from build123d import *

# Parameters (mm, degrees)
ESQUISSE1_W                  = 340
ESQUISSE1_H                  = 100.00000000000001
BOSS_EXTRU_1_DEPTH           = 10
ENL_V_MAT_EXTRU_1_DEPTH      = 355.54195802471673
ENL_V_MAT_EXTRU_1_DEPTH_BACK = 355.54195802471673
ESQUISSE2_R                  = 3.0000000000000018
ESQUISSE2_R_2                = 6.0000000000000036
ESQUISSE2_R_3                = 5.000000000000005
ESQUISSE2_R_4                = 6.000000000000017
ESQUISSE2_R_5                = 2.9999999999999947
ESQUISSE2_R_6                = 21.000000000000014
ESQUISSE2_W                  = 22.00000000000003
ESQUISSE2_H                  = 20.000000000000007
ENL_V_MAT_EXTRU_2_DEPTH      = 355.54195802471673
ENL_V_MAT_EXTRU_2_DEPTH_BACK = 355.54195802471673
ESQUISSE3_R                  = 2.2500000000000093
ESQUISSE3_R_2                = 2.2499999999999964
ESQUISSE3_R_3                = 2.2500000000000027
ESQUISSE3_R_4                = 2.2500000000000138
ESQUISSE5_R                  = 27.500000000000032
ESQUISSE5_R_2                = 8.999999999999984
ESQUISSE5_R_3                = 7.5000000000000115
ESQUISSE5_R_4                = 18.99999999999999
ESQUISSE5_R_5                = 11.499999999999993
ESQUISSE5_R_6                = 14.999999999999998
ESQUISSE5_R_7                = 11.499999999999998
ESQUISSE5_R_8                = 10.5
ENL_V_MAT_EXTRU_3_DEPTH      = 8
ESQUISSE6_W                  = 5.2500000000000036
ESQUISSE6_H                  = 11.999999999999993
ESQUISSE6_W_2                = 5.250000000000007
ESQUISSE6_W_3                = 5.25
BOSS_EXTRU_2_DEPTH           = 2
ESQUISSE8_R                  = 2.0000000000000027
ESQUISSE8_R_2                = 2.0000000000000018
ESQUISSE8_R_3                = 1.9999999999999967
ENL_V_MAT_EXTRU_4_DEPTH      = 10
ESQUISSE9_R                  = 6.999999999999988
ESQUISSE9_R_2                = 7.000000000000015
ESQUISSE9_R_3                = 7.000000000000002
ENL_V_MAT_EXTRU_5_DEPTH      = 8
CONG_1_R                     = 2
ENL_V_MAT_EXTRU_6_DEPTH      = 355.49118478405074
ENL_V_MAT_EXTRU_6_DEPTH_BACK = 355.49118478405074
CONG_2_R                     = 1.5
CONG_3_R                     = 1


with BuildPart() as part:
    # Esquisse1 → Boss.-Extru.1 (new body)
    with BuildSketch(Plane.XY):
        with Locations((170, 50.00000000000001)):
            Rectangle(ESQUISSE1_W, ESQUISSE1_H)
    extrude(amount=BOSS_EXTRU_1_DEPTH)

    # Esquisse2 → Enlèv. mat.-Extru.1 (cut, two sides: drawn at the far end of the back side and taken through both)
    with BuildSketch(Plane.XY.offset(10).offset(-ENL_V_MAT_EXTRU_1_DEPTH_BACK)):
        with Locations((15.000000000000007, 50)):
            Circle(ESQUISSE2_R)
        with Locations((41.00000000000001, 49.99999999999999)):
            Circle(ESQUISSE2_R_2)
        with Locations((86, 49.99999999999999)):
            Circle(ESQUISSE2_R_3)
        with Locations((131, 50)):
            Circle(ESQUISSE2_R_4)
        with Locations((216.00000000000003, 50)):
            Circle(ESQUISSE2_R_5)
        with Locations((261, 50)):
            Circle(ESQUISSE2_R_5)
        with Locations((306, 50)):
            Circle(ESQUISSE2_R_6)
        with Locations((171, 50)):
            Rectangle(ESQUISSE2_W, ESQUISSE2_H)
    extrude(amount=ENL_V_MAT_EXTRU_1_DEPTH + ENL_V_MAT_EXTRU_1_DEPTH_BACK, mode=Mode.SUBTRACT)

    # Esquisse3 → Enlèv. mat.-Extru.2 (cut, two sides: drawn at the far end of the back side and taken through both)
    with BuildSketch(Plane.XY.offset(10).offset(-ENL_V_MAT_EXTRU_2_DEPTH_BACK)):
        with Locations((170, 80)):
            Circle(ESQUISSE3_R)
        with Locations((100, 80)):
            Circle(ESQUISSE3_R_2)
        with Locations((30, 80)):
            Circle(ESQUISSE3_R_3)
        with Locations(Location((310.00000000000006, 80, 0), (0, 0, 180))):
            Circle(ESQUISSE3_R_4)
        with Locations(Location((240.00000000000003, 80, 0), (0, 0, 180))):
            Circle(ESQUISSE3_R)
    extrude(amount=ENL_V_MAT_EXTRU_2_DEPTH + ENL_V_MAT_EXTRU_2_DEPTH_BACK, mode=Mode.SUBTRACT)

    # Esquisse5 → Enlèv. mat.-Extru.3 (cut)
    with BuildSketch(Plane(origin=(0, 0, 0), x_dir=(-1, 0, 0), z_dir=(0, 0, -1))):
        with Locations((-306, 50)):
            Circle(ESQUISSE5_R)
        with Locations((-261, 50)):
            Circle(ESQUISSE5_R_2)
        with Locations((-216.00000000000003, 50)):
            Circle(ESQUISSE5_R_3)
        with Locations((-171, 50)):
            Circle(ESQUISSE5_R_4)
        with Locations((-131, 50)):
            Circle(ESQUISSE5_R_5)
        with Locations((-86, 49.99999999999999)):
            Circle(ESQUISSE5_R_6)
        with Locations((-41.00000000000001, 49.99999999999999)):
            Circle(ESQUISSE5_R_7)
        with Locations((-15.000000000000007, 50)):
            Circle(ESQUISSE5_R_8)
    extrude(amount=-ENL_V_MAT_EXTRU_3_DEPTH, mode=Mode.SUBTRACT)

    # Esquisse6 → Boss.-Extru.2 (add)
    with BuildSketch(Plane.XY.offset(10)):
        with Locations((33.12500000000001, 50)):
            Rectangle(ESQUISSE6_W, ESQUISSE6_H)
        with Locations((48.875000000000014, 50)):
            Rectangle(ESQUISSE6_W_2, ESQUISSE6_H)
        with Locations((123.12499999999997, 50)):
            Rectangle(ESQUISSE6_W_3, ESQUISSE6_H)
        with Locations((138.87500000000003, 50)):
            Rectangle(ESQUISSE6_W_3, ESQUISSE6_H)
    extrude(amount=-BOSS_EXTRU_2_DEPTH)

    # Esquisse8 → Enlèv. mat.-Extru.4 (cut)
    with BuildSketch(Plane.XY.offset(10)):
        with Locations((5, 90)):
            Circle(ESQUISSE8_R)
        with Locations(Location((5.00000000000001, 10.000000000000009, 0), (0, 0, 180))):
            Circle(ESQUISSE8_R_2)
        with Locations((335, 10.000000000000009)):
            Circle(ESQUISSE8_R_3)
        with Locations(Location((335, 90, 0), (0, 0, 180))):
            Circle(ESQUISSE8_R_3)
    extrude(amount=-ENL_V_MAT_EXTRU_4_DEPTH, mode=Mode.SUBTRACT)

    # Esquisse9 → Enlèv. mat.-Extru.5 (cut)
    with BuildSketch(Plane(origin=(0, 0, 0), x_dir=(-1, 0, 0), z_dir=(0, 0, -1))):
        with Locations((-310.00000000000006, 80)):
            Circle(ESQUISSE9_R)
        with Locations((-240.00000000000003, 80)):
            Circle(ESQUISSE9_R_2)
        with Locations((-170, 80)):
            Circle(ESQUISSE9_R_2)
        with Locations((-100, 80)):
            Circle(ESQUISSE9_R_3)
        with Locations((-30, 80)):
            Circle(ESQUISSE9_R_3)
    extrude(amount=-ENL_V_MAT_EXTRU_5_DEPTH, mode=Mode.SUBTRACT)

    # Congé1
    cong_1_edges = [part.edges().sort_by_distance(p)[0] for p in [
        (303.5061116987467, 77.38668510683382, 4),
        (315.5823162488517, 75.77652450015313, 4),
    ]]
    fillet(cong_1_edges, radius=CONG_1_R)

    # Esquisse10 → Enlèv. mat.-Extru.6 (cut, two sides: drawn at the far end of the back side and taken through both)
    with BuildSketch(Plane(origin=(0, 0, 8), x_dir=(-1, 0, 0), z_dir=(0, 0, -1)).offset(-ENL_V_MAT_EXTRU_6_DEPTH_BACK)):
        Polygon((-314.13172798364525, 65.90990257669736), (-321.90990257669733, 58.13172798364529), (-330.39518395093586, 66.61700935788389), (-322.6170093578838, 74.39518395093592), align=None)
        Polygon((-290.09009742330267, 41.8682720163547), (-281.60481604906414, 33.382990642116134), (-289.3829906421162, 25.60481604906408), (-297.86827201635475, 34.09009742330265), align=None)
    extrude(amount=ENL_V_MAT_EXTRU_6_DEPTH + ENL_V_MAT_EXTRU_6_DEPTH_BACK, mode=Mode.SUBTRACT)

    # Congé2
    cong_2_edges = [part.edges().sort_by_distance(p)[0] for p in [
        (281.60481604906414, 33.382990642116134, 5),
        (295.55817664855954, 31.780002055507403, 9),
        (289.3829906421162, 25.60481604906408, 5),
        (287.78000205550745, 39.55817664855947, 9),
        (330.39518395093586, 66.61700935788389, 5),
        (324.21999794449255, 60.44182335144051, 9),
        (316.44182335144046, 68.21999794449256, 9),
        (322.6170093578838, 74.39518395093592, 5),
    ]]
    fillet(cong_2_edges, radius=CONG_2_R)

    # Congé3
    # the kernel refuses this fillet: 1 mm, written as the material it takes off along each edge
    with BuildSketch(Plane(origin=(328.9416461797837, 65.16347158673169, 8), x_dir=(0.5395485077638712, -0.8419545164495408, 0), z_dir=(0, 0, -1))) as cong_3_piece_1:
        with BuildLine():
            CenterArc((0.7917838484009534, -0.9999000393817246), CONG_3_R, 90.81013186536997, 71.06099512229089)
            Line((-0.15857520364130714, -0.688744656652602), (-0.2536111088455419, -0.6576291183796682))
            ThreePointArc((-0.2536111088455419, -0.6576291183796682), (-0.216495562393325, -0.5213782577373202), (-0.09768701566509973, 0.02138333394130856))
            Line((-0.09768701566509973, 0.02138333394130856), (0.00141389972929694, 0.09999000393815428))
            ThreePointArc((0.00141389972929694, 0.09999000393815428), (0.3888224255540418, 0.09725108299714401), (0.7762309513787835, 0.09999000393816994))
            Line((0.7762309513787835, 0.09999000393816994), (0.7776448511080656, -5e-17))
        make_face()
    extrude(amount=9.944112127770163, mode=Mode.SUBTRACT)
    with BuildSketch(Plane(origin=(321.1634715867316, 72.94164617978372, 8), x_dir=(0.7147000811371469, 0.6994310502276516, 0), z_dir=(0, 0, -1))) as cong_3_piece_2:
        with BuildLine():
            CenterArc((0.7967561378121499, -0.9959424723360712), CONG_3_R, 95.16315700004625, 71.0609951222958)
            Line((-0.17447860578954866, -0.7578184021101204), (-0.27160208014971443, -0.7340059950875214))
            ThreePointArc((-0.27160208014971443, -0.7340059950875214), (-0.18201092031799704, -0.35708917183648514), (-0.09775794201756788, 0.02105670374221132))
            Line((-0.09775794201756788, 0.02105670374221132), (0.00107968352981501, 0.09999417124750024))
            ThreePointArc((0.00107968352981501, 0.09999417124750024), (0.5566601276180686, 0.093995311039016), (0.6977647438705182, 0.09959424723359925))
            Line((0.6977647438705182, 0.09959424723359925), (0.7067639615015904, -4e-17))
        make_face()
    extrude(amount=9.94411212777035, mode=Mode.SUBTRACT)
    with BuildSketch(Plane(origin=(283.0583538202163, 34.836528413268304, 8), x_dir=(-0.6994310502276408, -0.7147000811371573, 0), z_dir=(0, 0, -1))) as cong_3_piece_3:
        with BuildLine():
            CenterArc((0.7967561378121149, 0.9959424723360829), CONG_3_R, 193.7758478776647, 71.06099512228826)
            Line((-0.17447860578955895, 0.7578184021100173), (-0.27160208014972437, 0.7340059950874168))
            ThreePointArc((-0.27160208014972437, 0.7340059950874168), (-0.18201092031802182, 0.3570891718364219), (-0.09775794201756777, -0.02105670374219269))
            Line((-0.09775794201756777, -0.02105670374219269), (0.00107968352983153, -0.09999417124749502))
            ThreePointArc((0.00107968352983153, -0.09999417124749502), (0.5566601276181505, -0.09399531103902689), (0.6977647438704697, -0.09959424723361945))
            Line((0.6977647438704697, -0.09959424723361945), (0.7067639615015402, 5e-17))
        make_face()
    extrude(amount=9.944112127770104, mode=Mode.SUBTRACT)
    with BuildSketch(Plane(origin=(290.8365284132684, 27.05835382021624, 8), x_dir=(-0.7147000811371251, -0.6994310502276738, 0), z_dir=(0, 0, -1))) as cong_3_piece_4:
        with BuildLine():
            CenterArc((0.7967561378121253, -0.9959424723360709), CONG_3_R, 95.16315700004816, 71.0609951222958)
            Line((-0.17447860578957813, -0.7578184021101529), (-0.27160208014974474, -0.7340059950875569))
            ThreePointArc((-0.27160208014974474, -0.7340059950875569), (-0.18201092031804894, -0.35708917183650773), (-0.0977579420175735, 0.02105670374221336))
            Line((-0.0977579420175735, 0.02105670374221336), (0.00107968352981438, 0.09999417124749772))
            ThreePointArc((0.00107968352981438, 0.09999417124749772), (0.5566601276180955, 0.09399531103900281), (0.6977647438704596, 0.0995942472335964))
            Line((0.6977647438704596, 0.0995942472335964), (0.7067639615015323, -4e-17))
        make_face()
    extrude(amount=9.944112127770445, mode=Mode.SUBTRACT)


solid = part.part
Design review of the part built by this model. Coordinates are the model's own, in mm. A direction names the side the tool comes from. Round coordinates to 2 decimals unless told otherwise and drop trailing zeros. Answer as CSV lines item,"result". Start each with the question number.
1) Add section A-A (z = 3.75). Give the number of separate pieces and of enclosed holes in the cut face, then the cut area to 3 significant figures.
2) The part is to be moulded in two halves that separate along Y. For faces 4 (the face through (340, 49, 5)), 5 (the face through (297, 71, 8)), say which applies: +Y half, -Y half, draft (parallel to the pull), parting line (faces both ways), or undercut.
3) For pin 1 Ø5 at (x, y) = (170, 80) entering from -Z, flat-tipped, find the tip position at first contact; note if it passes through.
4) Wall thickness on line 1 along X through (y, z) = (90.5, 7.5); line 2 along Y through (x, z) = (170, 9.1); line 3 along X through (y, z) = (8.5, 2.25): over which ranges is each line inside the solid? List them lowest first. Write a range as [from, to].
5) Tool access review of faces 1 (the face through (285.454, 29.534, 5.07)), 2 (the face through (36, 45, 8)), 3 (the face through (0, 49, 5)): name each direction out of +Z, -Z, +X, -X, +Y, -Y from which nothing blocks a thin tool from reaching the whole face with its end or side.
Resolved:
1,separate pieces,"1"
1,enclosed holes,"16"
1,area,"27,400 mm^2"
2,face 4,"draft"
2,face 5,"undercut"
3,pin 1,"z = 8"
4,line 1,"[0, 3.06], [6.94, 333.06], [336.94, 340]"
4,line 2,"[0, 40], [60, 77.75], [82.25, 100]"
4,line 3,"[0, 3.68], [6.32, 333.68], [336.32, 340]"
5,face 1,"+Z, -Z"
5,face 2,"-Z"
5,face 3,"+Z, -Z, -X, +Y, -Y"
